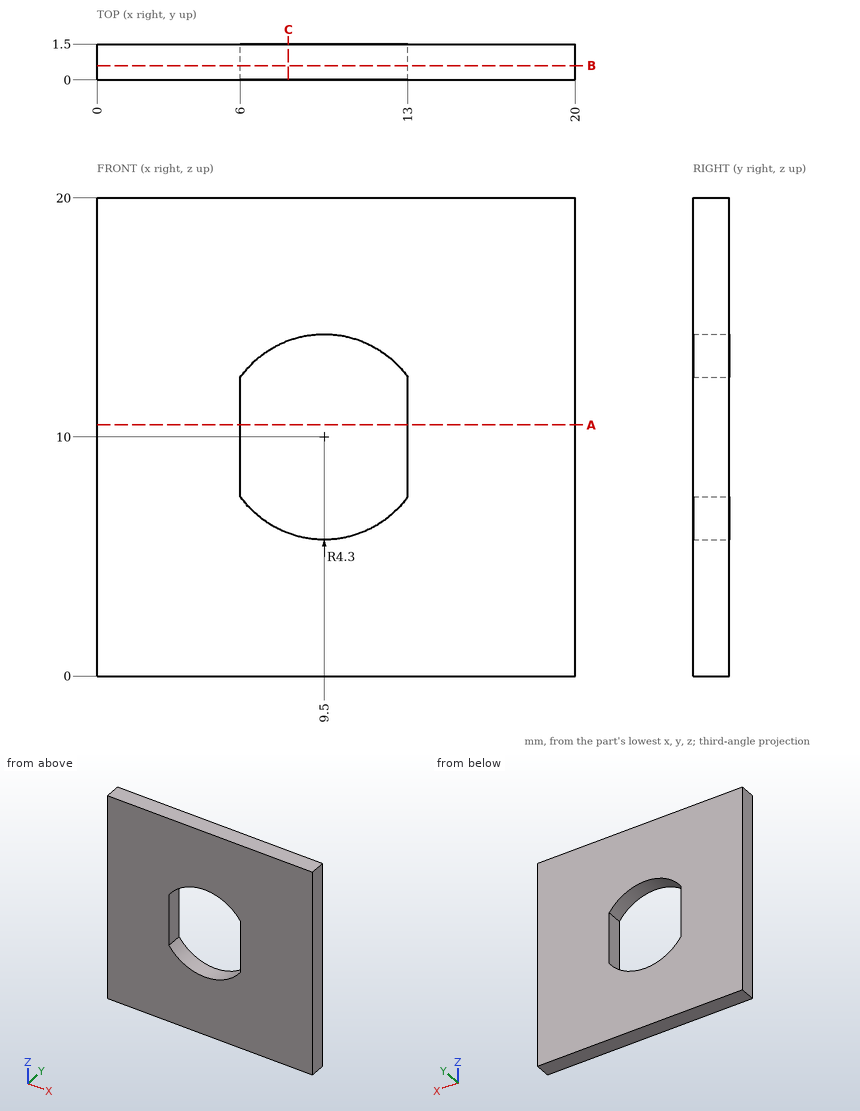
Check sheet for the drawn part. Datum: minimum x, y, z corner. Units: mm. Round coordinates to 2 decimals unless told otherwise and drop trailing zeros. Order: outer loops, then holes, each group sorted by start corner. A loop starts at its lowest first (then second) coordinate and runs counter-clockwise, first axis right, second up. Notation, with made-up numbers: (-37, 58.25) -> (-27, 58.25) arc R32 cw to (-27, 86.25) -> close; hole circle Ø5 at (80.25, 71). An arc over 180 degrees is marked (long way). Return JSON: item names as keys, results as strings. Group by question number.
Q1. Material ranges on probe 1 along X at (y, z) = (0.9, 10.5); probe 2 along Z at (x, y) = (12.75, 1.1); probe 3 along X at (y, z) = (1.25, 13.25), recorded low to high. Write a range as from..to.
Q2. Section check C-C, the plane x = 8. Record the boundary of the cut face in (y, z), plus the area to 3 significant figures.
Q3. Section check A-A, the plane z = 10.5. Record the boundary of the cut face in (x, y), plus the area to 3 significant figures.
Q4. Section check B-B, the plane y = 0.6. Record the boundary of the cut face in (x, z), plus the area to 3 significant figures.
Q5. Gauge pin test, flat end, axial feed: pin 1 (2 mm diameter, centred on x = 12.5, z = 8, fed in from -Y). Record the tip position at first contact, or that the pin passes through.
Numbers:
{
 "1": {"probe 1": "0..6, 13..20", "probe 2": "0..7.18, 12.82..20", "probe 3": "0..6.68, 12.32..20"},
 "2": {"outline": "(0, 0) -> (1.5, 0) -> (1.5, 5.97) -> (0, 5.97) -> close; (0, 14.03) -> (1.5, 14.03) -> (1.5, 20) -> (0, 20) -> close", "area": "17.9 mm^2"},
 "3": {"outline": "(0, 0) -> (6, 0) -> (6, 1.5) -> (0, 1.5) -> close; (13, 0) -> (20, 0) -> (20, 1.5) -> (13, 1.5) -> close", "area": "19.5 mm^2"},
 "4": {"outline": "(0, 0) -> (20, 0) -> (20, 20) -> (0, 20) -> close; hole (6, 7.5) arc R4.3 ccw to (13, 7.5) -> (13, 12.5) arc R4.3 ccw to (6, 12.5) -> close", "area": "347 mm^2"},
 "5": {"pin 1": "y = 0"}
}
